Could you check a few things on this model? Use its own coordinates, in mm. A direction names the side the tool comes from. Coordinates: 2 decimals unless noted, no trailing zeros. Loops run counter-clockwise (first coordinate to the right, second up) from the corner with the lowest first, then second, coordinate; pieces in that order, holes last. Notation, with made-up numbers: (-18.5, -34) -> (-6.5, -34) arc R22 cw to (-6.5, -26) -> close; hole circle Ø9 at (14, 7.5). An arc over 180 degrees is marked (long way). One line per question, with ' | ' between items.
```python
from build123d import *

# Parameters (mm, degrees)
F1_DEPTH = 63.5
F2_R     = 3.175
F3_DEPTH = 12.7
F6_DEPTH = 12.7


# Not quite as in the source:
# - a pattern or mirror of a feature is missing from the dataset's text; its kind, count and spacing are read off the source's solid


with BuildPart() as f1:
    # F0 (on Top) → F1 (new body, symmetric)
    with BuildSketch(Plane.XY):
        Polygon((-346.075, -406.4), (346.075, -406.4), (346.075, -393.7), (346.075, 406.4), (-290.28644, 406.4), (-294.2266940207, 406.4), (-346.075, 406.4), (-346.075, 393.7), align=None)
        Polygon((-276.225, 393.7), (-276.225, 383.1179738045), (-276.225, -393.7), (-333.375, -393.7), (-333.375, 393.7), align=None, mode=Mode.SUBTRACT)
        Polygon((-263.525, -393.7), (-263.525, 383.1179738045), (-263.525, 393.7), (263.525, 393.7), (263.525, 383.1179738045), (263.525, -393.7), align=None, mode=Mode.SUBTRACT)
        Polygon((333.375, 393.7), (333.375, -393.7), (276.225, -393.7), (276.225, 383.1179738045), (276.225, 393.7), align=None, mode=Mode.SUBTRACT)
    extrude(amount=F1_DEPTH, both=True)

    # F2 (on face) → F3 (cut)
    with BuildSketch(Plane(origin=(263.525, 0, 0), x_dir=(0, -1, 0), z_dir=(-1, 0, 0))):
        Circle(F2_R)
        with Locations((-279.4, 0)):
            Circle(F2_R)
        with Locations((279.4, 0)):
            Circle(F2_R)
    f3 = extrude(amount=-F3_DEPTH, mode=Mode.SUBTRACT)

    # F3_copies: F3 across plane
    add(f3.mirror(Plane(origin=(0, 0, 0), x_dir=(0, 0, -1), z_dir=(-1, 0, 0))), mode=Mode.SUBTRACT)

    # F5 (on mid) → F6 (join, symmetric)
    with BuildSketch(Plane.YZ.offset(339.725)):
        Polygon((-215.9, 63.5), (-203.2, 63.5), (-190.5, 63.5), (-190.5, 114.3), (-215.9, 114.3), align=None)
        Polygon((190.5, 63.5), (203.2, 63.5), (215.9, 63.5), (215.9, 114.3), (190.5, 114.3), align=None)
    f6 = extrude(amount=F6_DEPTH, both=True)

    # F6_copies: F6 across plane
    add(f6.mirror(Plane(origin=(0, 0, 0), x_dir=(0, 0, -1), z_dir=(-1, 0, 0))))

    # F6_copies1: F6 across plane
    add(f6.mirror(Plane(origin=(304.8, 0, 0), x_dir=(0, 0, -1), z_dir=(-1, 0, 0))))

    # F6_copies2: F6 across plane
    add(f6.mirror(Plane(origin=(34.925, 0, 0), x_dir=(0, 0, -1), z_dir=(-1, 0, 0))))


solid = f1.part
```
Q1. For faces 1 (the face through (-340, 215.9, 89)), 2 (the face through (340, 190.5, 89)), 3 (the face through (327.025, -203, 89)), which set-ups out of +Z, -Z, +X, -X, +Y, -Y let a thin tool reach every point of the face, with its end or its side?
Values follow:
face 1: +Z, +X, -X, +Y | face 2: +Z, +X, -X | face 3: +Z, -Z, +Y, -Y
Q2. Imagine slicing it at B-B on y = 153. Write out the boundary of the cut face in (x, z) (3 decimals), plus the area to 3 significant figures.
Values follow:
outline: (-346.075, -63.5) -> (-333.375, -63.5) -> (-333.375, 63.5) -> (-346.075, 63.5) -> close; (-276.225, -63.5) -> (-263.525, -63.5) -> (-263.525, 63.5) -> (-276.225, 63.5) -> close; (263.525, -63.5) -> (276.225, -63.5) -> (276.225, 63.5) -> (263.525, 63.5) -> close; (333.375, -63.5) -> (346.075, -63.5) -> (346.075, 63.5) -> (333.375, 63.5) -> close | area: 6,450 mm2
Q3. For pin 1 (12 mm diameter, centred on y = 186, z = 28, fed in from +X) (3 decimals); pin 2 (4 mm diameter, centred on y = -279.4, z = 0, fed in from -X) (3 decimals); pin 3 (7.5 mm diameter, centred on x = 342.5, z = 86, fed in from -Y), each with a flat end and sliding along its axis, tell me the tip position at first contact or that it passes through.
Values follow:
pin 1: stops at x = 346.075 | pin 2: stops at x = -346.075 | pin 3: stops at y = -215.9
Q4. Imagine slicing it at C-C on z = -28.5. Write out the boundary of the cut face in (x, y) (3 decimals), plus the area to 3 significant figures.
Values follow:
outline: (-346.075, -406.4) -> (346.075, -406.4) -> (346.075, 406.4) -> (-346.075, 406.4) -> close; hole (-333.375, -393.7) -> (-276.225, -393.7) -> (-276.225, 393.7) -> (-333.375, 393.7) -> close; hole (-263.525, -393.7) -> (263.525, -393.7) -> (263.525, 393.7) -> (-263.525, 393.7) -> close; hole (276.225, -393.7) -> (333.375, -393.7) -> (333.375, 393.7) -> (276.225, 393.7) -> close | area: 57,600 mm2
Q5. We'd pull the mould along Y, two halves only. Please class faces 4 (the face through (340, 215.9, 89)), 5 (the face through (-340, -190.5, 89)), 6 (the face through (-327.025, -203, 89)): released by +Y, released by -Y, zero draft, split by the parting line, or undercut.
Values follow:
face 4: released by +Y | face 5: undercut | face 6: zero draft
Q6. Please list where these lines run through material, in increasing order: L1, parallel to X at y = -273.5, z = 40 (3 decimals); L2, parallel to Z at x = -273.5, y = 279.4 (3 decimals); L3, parallel to Y at x = -138.5, z = -39. Write a range as [from, to].
Values follow:
L1: x = [-346.075, -333.375], [-276.225, -263.525], [263.525, 276.225], [333.375, 346.075] | L2: z = [-63.5, -3.175], [3.175, 63.5] | L3: y = [-406.4, -393.7], [393.7, 406.4]
Q7. Imagine slicing it at A-A on x = 91. Write out the boundary of the cut face in (y, z), plus the area to 3 significant figures.
Values follow:
outline: (-406.4, -63.5) -> (-393.7, -63.5) -> (-393.7, 63.5) -> (-406.4, 63.5) -> close; (393.7, -63.5) -> (406.4, -63.5) -> (406.4, 63.5) -> (393.7, 63.5) -> close | area: 3,230 mm2
